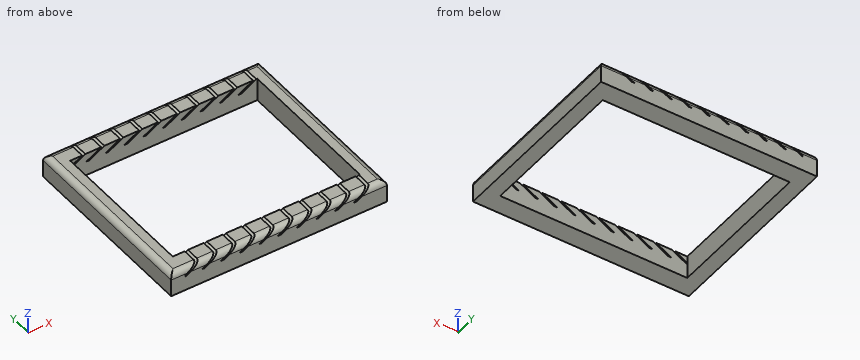
from build123d import *

# Parameters (mm, degrees)
F0_W     = 75
F0_H     = 65
F1_DEPTH = 8
F2_R     = 2
F3_W     = 65
F3_H     = 52
F4_DEPTH = 8.001
F7_DEPTH = 6.501
F8_DEPTH = 6.501


with BuildPart() as f1:
    # F0 (on Top) → F1 (new body)
    with BuildSketch(Plane.XY):
        Rectangle(F0_W, F0_H)
    extrude(amount=F1_DEPTH)

    # F2
    f2_edges = [f1.edges().sort_by_distance(p)[0] for p in [
        (0, -32.5, 8),
        (37.5, 0, 8),
        (0, 32.5, 8),
        (-37.5, 0, 8),
    ]]
    fillet(f2_edges, radius=F2_R)

    # F3 (on face) → F4 (cut, through all)
    with BuildSketch(Plane.XY.offset(8)):
        Rectangle(F3_W, F3_H)
    extrude(amount=-F4_DEPTH, mode=Mode.SUBTRACT)

    # F5 (on face) → F7 (cut, through all)
    with BuildSketch(Plane.XZ.offset(-26)):
        Polygon((-27.241326, 8), (-28.341326, 8), (-32.5, 5.598989), (-32.5, 5.021638), (-32.4, 5.021638), align=None)
        Polygon((-20.641326, 8), (-21.741326, 8), (-26.9, 5.021638), (-25.8, 5.021638), align=None)
        Polygon((-14.041326, 8), (-15.141326, 8), (-20.3, 5.021638), (-19.2, 5.021638), align=None)
        Polygon((-7.441326, 8), (-8.541326, 8), (-13.7, 5.021638), (-12.6, 5.021638), align=None)
        Polygon((-0.841326, 8), (-1.941326, 8), (-7.1, 5.021638), (-6, 5.021638), align=None)
        Polygon((5.758674, 8), (4.658674, 8), (-0.5, 5.021638), (0.6, 5.021638), align=None)
        Polygon((12.358674, 8), (11.258674, 8), (6.1, 5.021638), (7.2, 5.021638), align=None)
        Polygon((13.8, 5.021638), (18.958674, 8), (17.858674, 8), (12.7, 5.021638), align=None)
        Polygon((20.4, 5.021638), (25.558674, 8), (24.458674, 8), (19.3, 5.021638), align=None)
        Polygon((27, 5.021638), (32.158674, 8), (31.058674, 8), (25.9, 5.021638), align=None)
    extrude(amount=-F7_DEPTH, mode=Mode.SUBTRACT)

    # F6 (on face) → F8 (cut, through all)
    with BuildSketch(Plane(origin=(0, -26, 0), x_dir=(-1, 0, 0), z_dir=(0, 1, 0))):
        Polygon((32.5, 5.598989), (28.341326, 8), (27.241326, 8), (32.45, 4.992771), align=None)
        Polygon((26.9, 5.021638), (21.741326, 8), (20.641326, 8), (25.8, 5.021638), align=None)
        Polygon((20.3, 5.021638), (15.141326, 8), (14.041326, 8), (19.2, 5.021638), align=None)
        Polygon((13.7, 5.021638), (8.541326, 8), (7.441326, 8), (12.6, 5.021638), align=None)
        Polygon((7.1, 5.021638), (1.941326, 8), (0.841326, 8), (6, 5.021638), align=None)
        Polygon((0.5, 5.021638), (-4.658674, 8), (-5.758674, 8), (-0.6, 5.021638), align=None)
        Polygon((-11.258674, 8), (-12.358674, 8), (-7.2, 5.021638), (-6.1, 5.021638), align=None)
        Polygon((-17.858674, 8), (-18.958674, 8), (-13.8, 5.021638), (-12.7, 5.021638), align=None)
        Polygon((-24.458674, 8), (-25.558674, 8), (-20.4, 5.021638), (-19.3, 5.021638), align=None)
        Polygon((-31.058674, 8), (-32.158674, 8), (-27, 5.021638), (-25.9, 5.021638), align=None)
    extrude(amount=-F8_DEPTH, mode=Mode.SUBTRACT)


solid = f1.part
Model file for the job. Use its own axes, mm. Coordinates: 2 decimals unless noted, no trailing zeros. Write each loop counter-clockwise with the first axis right and the second up, starting at its lowest first coordinate (ties: lowest second). Pieces come first, ordered by that corner, then holes. Notation, with made-up numbers: (14, 88) -> (53, 88) arc R11 ccw to (53, 99) -> close; hole circle Ø7 at (41.25, -38.75). An arc over 180 degrees is marked (long way). One line per item, written item: value. Start each with the question number.
1) Flat gauge pins, fed straight in: pin 1 Ø1.5 at (x, z) = (-3, 7) entering from +Y; pin 2 Ø1.2 at (x, z) = (-31, 7.5) entering from +Y. Where does each tip first touch, or does it go through?
2) Slice it at B-B on z = 1.5. Write the cut outline in (x, y).
3) Slice it at C-C on x = -3.5. Write the cut outline in (y, z), then the cut area to 3 significant figures.
4) Probe probe 1 along X at (y, z) = (-16.5, 1.5); probe 2 along Y at (x, z) = (-28.5, 1.5); probe 3 along X at (y, z) = (8, 7.25). List the from-to ranges inside material, lowest first.
5) Slice it at A-A on y = -5. Write the cut outline in (x, z), then the cut area to 3 significant figures.
Answers follow:
1. pin 1: y = 32.48
1. pin 2: y = 32.29
2. outline: (-37.5, -32.5) -> (37.5, -32.5) -> (37.5, 32.5) -> (-37.5, 32.5) -> close; hole (-32.5, -26) -> (32.5, -26) -> (32.5, 26) -> (-32.5, 26) -> close
3. outline: (-32.5, 0) -> (-26, 0) -> (-26, 6.47) -> (-32.45, 6.47) arc R2 ccw to (-32.5, 6) -> close; (-32.17, 7.1) -> (-26, 7.1) -> (-26, 8) -> (-30.5, 8) arc R2 ccw to start; (26, 0) -> (32.5, 0) -> (32.5, 6) arc R2 ccw to (32.45, 6.47) -> (26, 6.47) -> close; (26, 7.1) -> (32.17, 7.1) arc R2 ccw to (30.5, 8) -> (26, 8) -> close
3. area: 94.2 mm2
4. probe 1: -37.5 to -32.5, 32.5 to 37.5
4. probe 2: -32.5 to -26, 26 to 32.5
4. probe 3: -37.06 to -32.5, 32.5 to 37.06
5. outline: (-37.5, 0) -> (-32.5, 0) -> (-32.5, 8) -> (-35.5, 8) arc R2 ccw to (-37.5, 6) -> close; (32.5, 0) -> (37.5, 0) -> (37.5, 6) arc R2 ccw to (35.5, 8) -> (32.5, 8) -> close
5. area: 78.3 mm2
